Verification items for this drawing (mm, ordinates from the low corner). A direction names the side the tool comes from. Round coordinates to 2 decimals unless told otherwise and drop trailing zeros. Order: outer loops, then holes, each group sorted by start corner. A loop starts at its lowest first (then second) coordinate and runs counter-clockwise, first axis right, second up. Notation, with made-up numbers: (74, 47) - (90, 47) arc R21 ccw to (90, 80) - close; hole circle Ø9 at (16, 36). An arc over 180 degrees is marked (long way). Use a Markdown table: item, result. Add a question column.
(1) Section check A-A on y = 50. Record the boundary of the cut face in (x, z).
(2) Section check D-D on z = 16. Record the boundary of the cut face in (x, y), then the cut area to 3 significant figures.
(3) Mould release check, pull along Y, two halves, no side actions. Record for the marked faces 1, 2 and 3: released by +Y, released by -Y, zero draft, split by the parting line, or undercut.
(4) Access from +Z, -Z, +X, -X, +Y, -Y to the whole of each face (thin tool, end or side, straight path). Record for the marked faces 4 and 5.
(5) Gauge pin test, flat ends, axial feed: P1, Ø8, axis at x = 52, y = 49.5, coming from the +Z side; P2, Ø5, axis at y = 58.5, z = 10.5, coming from the -X side; P3, Ø12, axis at x = 88, z = 32, coming from the -Y side. Record the tip position at first contact, or that the pin passes through.
(6) Section check C-C on z = 6.5. Record the boundary of the cut face in (x, y), then the cut area to 3 significant figures.
(7) Thickness scan on line 1 along Y through (x, z) = (50, 6); line 2 along X through (y, z) = (51, 22). Record the ranges inside material, lowest first. Write a range as [from, to].
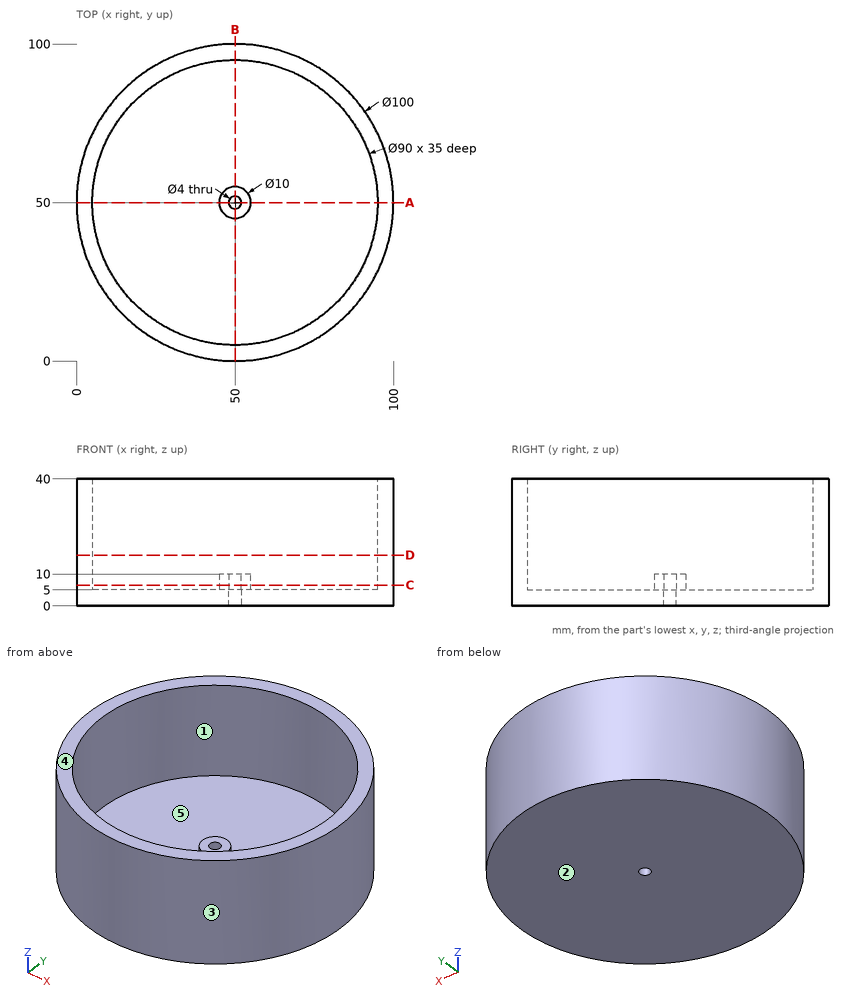
Check sheet entries:
| question | item | result |
|---|---|---|
| 1 | outline | (0, 0) - (48, 0) - (48, 10) - (45, 10) - (45, 5) - (5, 5) - (5, 40) - (0, 40) - close; (52, 0) - (100, 0) - (100, 40) - (95, 40) - (95, 5) - (55, 5) - (55, 10) - (52, 10) - close |
| 2 | outline | circle Ø100 at (50, 50); hole circle Ø90 at (50, 50) |
| 2 | area | 1,490 mm2 |
| 3 | face 1 | undercut |
| 3 | face 2 | zero draft |
| 3 | face 3 | split by the parting line |
| 4 | face 4 | +Z, +X, -X, +Y, -Y |
| 4 | face 5 | +Z |
| 5 | P1 | stops at z = 10 |
| 5 | P2 | stops at x = 0.36 |
| 5 | P3 | stops at y = 11.58 |
| 6 | outline | circle Ø100 at (50, 50); circle Ø10 at (50, 50); hole circle Ø90 at (50, 50); hole circle Ø4 at (50, 50) |
| 6 | area | 1,560 mm2 |
| 7 | line 1 | y = [0, 5], [45, 48], [52, 55], [95, 100] |
| 7 | line 2 | x = [0.01, 5.01], [94.99, 99.99] |
